Autodesk Inventor part; units mm, degrees
ref_plane "YZ Plane" through (0, 0, 0) normal (1, 0, 0) x (0, 1, 0)
ref_plane "XZ Plane" through (0, 0, 0) normal (0, 1, 0) x (-1, 0, 0)
ref_plane "XY Plane" through (0, 0, 0) normal (0, 0, 1) x (1, 0, 0)
sketch "Sketch1" plane through (0, 0, 0) normal (0, 0, 1) x (1, 0, 0)
  circle A0 centre (0, 0) radius 20
  circle A1 centre (0, 0) radius 15
  circle A2 centre (0, 0) radius 13
  circle A3 centre (0, 0) radius 14
  dimension "d0" = 40
  dimension "d1" = 5
  dimension "d2" = 2
  dimension "d3" = 1
extrude "Extrusion1" add sketch "Sketch1" along normal blind 40 contours A1
sketch "Sketch2" plane through (0, 0, 40) normal (0, 0, 1) x (1, 0, 0)
  point P0 (0, 0)
sketch "Sketch3" plane through (0, 0, 40) normal (0, 0, 1) x (1, 0, 0)
  circle A0 centre (0, 0) radius 20
  dimension "d6" = 40
extrude "Extrusion2" add sketch "Sketch3" along normal blind 5
sketch "Sketch4" plane through (0, 0, 0) normal (0, 0, -1) x (-1, 0, 0)
  circle A0 centre (0, 0) radius 17.5
  dimension "d9" = 35
extrude "Extrusion3" add sketch "Sketch4" along normal blind 3
sketch "Sketch5" plane through (0, 0, 45) normal (0, 0, 1) x (1, 0, 0)
  point P0 (0, 0)
sketch "Sketch6" plane through (0, 0, 45) normal (0, 0, 1) x (1, 0, 0)
  circle A0 centre (0, 0) radius 15
properties part number "weird_cylinder"
Check sheet for the modelled part. Datum: model origin and axes. Units: mm. A direction names the side the tool comes from. Coordinates: 2 decimals unless noted, no trailing zeros. Order: outer loops, then holes, each group sorted by start corner. A loop starts at its lowest first (then second) coordinate and runs counter-clockwise, first axis right, second up. Notation, with made-up numbers: (-17.75, 9) -> (23.25, 9) arc R9 cw to (23.25, 19) -> close; hole circle Ø3 at (61, -15). An arc over 180 degrees is marked (long way). Write item = value, one per line. Start each with the question number.
1) Go/stop test with flat-tipped pins: P1, Ø8, axis at y = 15.5, z = 32, coming from the -X side; P2, Ø10, axis at x = -4.5, z = 35.5, coming from the +Y side; P3, Ø5, axis at y = 3.5, z = 20.5, coming from the -X side. Record where each tip stops, or that it passes through.
2) Cross-section at B-B (y = -10). Enter the section's corners in (x, z).
3) Mould release check, pull along Y, two halves, no side actions. Record for faces 4 (the cylindrical face through (12.932, 5.362, 19.72)), 5 (the flat face through (-13, 8, 0)), 6 (the flat face through (0, 0, 40)), 7 (the cylindrical face through (-14.985, -0.66, 19.72)): +Y half, -Y half, draft (parallel to the pull), parting line (faces both ways), or undercut.
4) Cross-section at C-C (z = 29.5). Enter the section's corners in (x, y), then the cut area to 3 significant figures.
5) Cross-section at A-A (x = 0). Enter the section's corners in (y, z).
6) Access from +Z, -Z, +X, -X, +Y, -Y to the whole of each face (thin tool, end or side, straight path). Record for faces 1 (the cylindrical face through (-4.336, 19.524, 42.465)), 2 (the flat face through (0, 0, 0)), 3 (the cylindrical face through (13.887, 10.648, -1.479)).
7) Material ranges on L1, parallel to Z at x = -5, y = 6; L2, parallel to Y at x = 0, z = 12.5; L3, parallel to X at y = 9.5, z = 24.5, recorded low to high.
Ans:
q1.P1 = -9.63
q1.P2 = 19.86
q1.P3 = -14.97
q2.outline = (-17.32, 40) -> (-11.18, 40) -> (-11.18, 0) -> (-14.36, 0) -> (-14.36, -3) -> (14.36, -3) -> (14.36, 0) -> (11.18, 0) -> (11.18, 40) -> (17.32, 40) -> (17.32, 45) -> (-17.32, 45) -> close; hole (-9.8, 0) -> (9.8, 0) -> (9.8, 40) -> (-9.8, 40) -> close
q3.face_4 = undercut
q3.face_5 = draft
q3.face_6 = undercut
q3.face_7 = parting line
q4.outline = circle Ø30 at (0, 0); hole circle Ø28 at (0, 0)
q4.area = 91.1 mm²
q5.outline = (-20, 40) -> (-15, 40) -> (-15, 0) -> (-17.5, 0) -> (-17.5, -3) -> (17.5, -3) -> (17.5, 0) -> (15, 0) -> (15, 40) -> (20, 40) -> (20, 45) -> (-20, 45) -> close; hole (-14, 0) -> (14, 0) -> (14, 40) -> (-14, 40) -> close
q6.face_1 = +Z, -Z
q6.face_2 = none
q6.face_3 = -Z
q7.L1 = -3 to 0, 40 to 45
q7.L2 = -15 to -14, 14 to 15
q7.L3 = -11.61 to -10.28, 10.28 to 11.61
